from build123d import *

# Parameters (mm, degrees)
F0_W     = 45.234501
F0_H     = 83.036979
F1_DEPTH = 36.576
F2_DEPTH = 36.576


with BuildPart() as f1:
    # F0 (on Top) → F1 (new body)
    with BuildSketch(Plane.XY):
        Polygon((232.690369, 341.347511), (-452.865685, 341.347511), (232.690369, -342.956906), (232.690369, -171.880802), (232.690369, -0.804697), align=None)
        with Locations((189.227968, 118.748626)):
            Rectangle(F0_W, F0_H, mode=Mode.SUBTRACT)
        Polygon((-31.388473, 320.019749), (51.648368, 320.17149), (51.731029, 274.937065), (-31.305811, 274.785323), align=None, mode=Mode.SUBTRACT)
    extrude(amount=F1_DEPTH)

    # F0 (on Top) → F2 (join)
    with BuildSketch(Plane.XY):
        Polygon((232.690369, 341.347511), (-452.865685, 341.347511), (232.690369, -342.956906), (232.690369, -171.880802), (232.690369, -0.804697), align=None)
        with Locations((189.227968, 118.748626)):
            Rectangle(F0_W, F0_H, mode=Mode.SUBTRACT)
        Polygon((-31.388473, 320.019749), (51.648368, 320.17149), (51.731029, 274.937065), (-31.305811, 274.785323), align=None, mode=Mode.SUBTRACT)
    extrude(amount=F2_DEPTH)


solid = f1.part
Geometry check sheet. Reference: the model listing, model coordinates, mm. A direction names the side the tool comes from. Round coordinates to 2 decimals unless told otherwise and drop trailing zeros. Loops run counter-clockwise (first coordinate to the right, second up) from the corner with the lowest first, then second, coordinate; pieces in that order, holes last.
Item 1: Cross-section at C-C on y = 109. Record the boundary of the cut face in (x, z).
Item 2: Cross-section at A-A on x = -19. Record the boundary of the cut face in (y, z), then the cut area to 3 significant figures.
Item 3: Thickness scan on line 1 (X direction, y = 286, z = 10.5); line 2 (X direction, y = 284.5, z = 24); line 3 (X direction, y = -226, z = 19). Record the ranges inside material, lowest first.
Item 4: Access from +Z, -Z, +X, -X, +Y, -Y to the whole of each face (thin tool, end or side, straight path). Record for faces 4 (the flat face through (189, 77.23, 18)), 5 (the flat face through (37, 156, 0)).
Item 5: Gauge pin test, flat ends, axial feed: pin 1 (2 mm diameter, centred on y = -81.5, z = 10, fed in from -X); pin 2 (1 mm diameter, centred on y = -50.5, z = 15, fed in from -X); pin 3 (12 mm diameter, centred on y = 52, z = 18.5, fed in from -X). Record the tip position at first contact, or that the pin passes through.
Item 6: Cross-section at B-B on z = 23. Record the boundary of the cut face in (x, y).
Item 7: Cross-section at D-D on x = -284. Record the boundary of the cut face in (y, z), then the cut area to 3 significant figures.
Item 8: Mould release check, pull along X, two halves, no side actions. Record for faces 1 (the flat face through (232.69, -6, 18)), 2 (the flat face through (189, 160.267, 18)), 3 (the flat face through (-114.9, 4, 18)): pulls with the +X half, pulls with the -X half, needs draft (parallel to the pull), parting line crosses it, or undercut.
Answer sheet:
1. outline: (-220.09, 0) - (166.61, 0) - (166.61, 36.58) - (-220.09, 36.58) - close; (211.85, 0) - (232.69, 0) - (232.69, 36.58) - (211.85, 36.58) - close
2. outline: (-91.73, 0) - (274.81, 0) - (274.81, 36.58) - (-91.73, 36.58) - close; (320.04, 0) - (341.35, 0) - (341.35, 36.58) - (320.04, 36.58) - close
2. area: 14,200 mm2
3. line 1: x = -397.42 to -31.33, 51.71 to 232.69
3. line 2: x = -395.91 to -31.32, 51.71 to 232.69
3. line 3: x = 115.52 to 232.69
4. face 4: +Z, -Z
4. face 5: -Z, +X, -X, +Y, -Y
5. pin 1: stops at x = -30.25
5. pin 2: stops at x = -60.8
5. pin 3: stops at x = -169
6. outline: (-452.87, 341.35) - (232.69, -342.96) - (232.69, 341.35) - close; hole (-31.39, 320.02) - (-31.31, 274.79) - (51.73, 274.94) - (51.65, 320.17) - close; hole (166.61, 77.23) - (211.85, 77.23) - (211.85, 160.27) - (166.61, 160.27) - close
7. outline: (172.79, 0) - (341.35, 0) - (341.35, 36.58) - (172.79, 36.58) - close
7. area: 6,170 mm2
8. face 1: pulls with the +X half
8. face 2: undercut
8. face 3: pulls with the -X half
